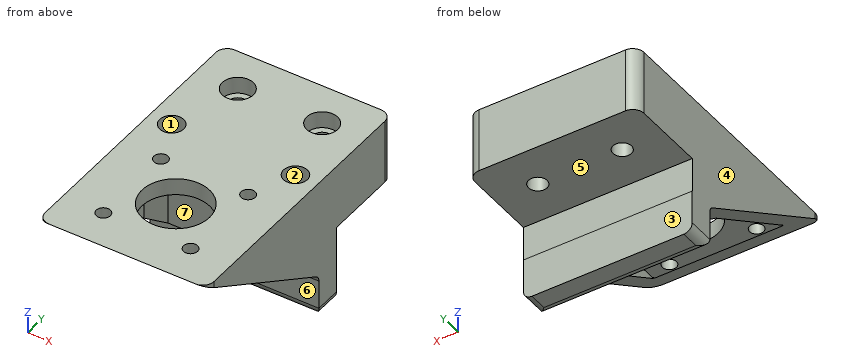
```python
from build123d import *

# Parameters (mm, degrees)
ESBO_O1_R                         = 12
ESBO_O1_R_2                       = 2.5
RESSALTO_EXTRUS_O1_DEPTH          = 6
RESSALTO_EXTRUS_O2_DEPTH          = 50
CORTE_EXTRUS_O1_DEPTH             = 61
ESBO_O5_R                         = 4.25
CORTE_EXTRUS_O2_DEPTH             = 15
REBAIXO_PARA_SHCS_M61_D           = 6.6
REBAIXO_PARA_SHCS_M61_CBORE_D     = 11
REBAIXO_PARA_SHCS_M61_CBORE_DEPTH = 6
CORTE_EXTRUS_O3_DEPTH             = 61
ESBO_O4_W                         = 60
ESBO_O4_H                         = 9.5
RESSALTO_EXTRUS_O3_DEPTH          = 15
FILETE1_R                         = 3


with BuildPart() as part:
    # Esboço1 → Ressalto-extrusão1 (new body)
    with BuildSketch(Plane.XY.offset(29.3)):
        with BuildLine():
            Line((-245.980789633, -100), (-193.980789633, -100))
            ThreePointArc((-193.980789633, -100), (-191.152362508, -98.828427125), (-189.980789633, -96))
            Line((-189.980789633, -96), (-189.980789633, -4))
            ThreePointArc((-189.980789633, -4), (-191.152362508, -1.171572875), (-193.980789633, 0))
            Line((-193.980789633, 0), (-245.980789633, 0))
            ThreePointArc((-245.980789633, 0), (-248.809216758, -1.171572875), (-249.980789633, -4))
            Line((-249.980789633, -4), (-249.980789633, -96))
            ThreePointArc((-249.980789633, -96), (-248.809216758, -98.828427125), (-245.980789633, -100))
        make_face()
        with Locations((-219.980789633, -71.15)):
            Circle(ESBO_O1_R, mode=Mode.SUBTRACT)
        with Locations((-235.480789633, -86.65)):
            Circle(ESBO_O1_R_2, mode=Mode.SUBTRACT)
        with Locations((-235.480789633, -55.65)):
            Circle(ESBO_O1_R_2, mode=Mode.SUBTRACT)
        with Locations((-204.480789633, -86.65)):
            Circle(ESBO_O1_R_2, mode=Mode.SUBTRACT)
        with Locations((-204.480789633, -55.65)):
            Circle(ESBO_O1_R_2, mode=Mode.SUBTRACT)
    extrude(amount=RESSALTO_EXTRUS_O1_DEPTH)

    # Esboço2 → Ressalto-extrusão2 (add)
    with BuildSketch(Plane(origin=(0, 0, 29.3), x_dir=(-1, 0, 0), z_dir=(0, 0, -1))):
        with BuildLine():
            Line((189.980789633, -4), (189.980789633, -96))
            ThreePointArc((189.980789633, -96), (191.152362508, -98.828427125), (193.980789633, -100))
            Line((193.980789633, -100), (245.980789633, -100))
            ThreePointArc((245.980789633, -100), (248.809216758, -98.828427125), (249.980789633, -96))
            Line((249.980789633, -96), (249.980789633, -4))
            ThreePointArc((249.980789633, -4), (248.809216758, -1.171572875), (245.980789633, 0))
            Line((245.980789633, 0), (193.980789633, 0))
            ThreePointArc((193.980789633, 0), (191.152362508, -1.171572875), (189.980789633, -4))
        make_face()
        Polygon((237.959216758, -48), (202.002362508, -48), (196.830789633, -53.171572875), (196.830789633, -89.128427125), (202.002362508, -94.3), (237.959216758, -94.3), (243.130789633, -89.128427125), (243.130789633, -53.171572875), align=None, mode=Mode.SUBTRACT)
    extrude(amount=RESSALTO_EXTRUS_O2_DEPTH)

    # Esboço3 → Corte-extrusão1 (cut, through all)
    with BuildSketch(Plane.ZY.offset(249.980789633)):
        Polygon((35.3, -100), (-20.7, -100), (-20.7, -31.056412858), (0, -31.056412858), (0, -39.485714286), align=None)
    extrude(amount=-CORTE_EXTRUS_O1_DEPTH, mode=Mode.SUBTRACT)

    # Esboço5 → Corte-extrusão2 (cut)
    with BuildSketch(Plane.XY.offset(35.3)):
        with Locations((-241.980789633, -40)):
            Circle(ESBO_O5_R)
        with Locations((-197.980789633, -40)):
            Circle(ESBO_O5_R)
    extrude(amount=-CORTE_EXTRUS_O2_DEPTH, mode=Mode.SUBTRACT)

    # Rebaixo para SHCS M61 (through all)
    with Locations(Plane.XY.offset(35.3)):
        with Locations((-234.980789633, -15), (-204.980789633, -15)):
            CounterBoreHole(REBAIXO_PARA_SHCS_M61_D / 2, REBAIXO_PARA_SHCS_M61_CBORE_D / 2, REBAIXO_PARA_SHCS_M61_CBORE_DEPTH)

    # Esboço10 → Corte-extrusão3 (cut, through all)
    with BuildSketch(Plane.ZY.offset(249.980789633)):
        Polygon((12.291276716, 1.7848e-05), (-27.708723284, 1.7848e-05), (-27.708723284, -29.999982152), (-21.235336221, -29.999982152), (-21.235336221, -31.532793492), (0, -31.532793492), (0, -29.999982152), (12.291276716, -29.999982152), align=None)
    extrude(amount=-CORTE_EXTRUS_O3_DEPTH, mode=Mode.SUBTRACT)

    # Esboço4 → Ressalto-extrusão3 (add)
    with BuildSketch(Plane(origin=(0, 0, 0), x_dir=(-1, 0, 0), z_dir=(0, 0, -1))):
        with Locations((219.980789633, -34.735714286)):
            Rectangle(ESBO_O4_W, ESBO_O4_H)
    extrude(amount=RESSALTO_EXTRUS_O3_DEPTH)

    # Filete1
    filete1_edges = [part.edges().sort_by_distance(p)[0] for p in [
        (-219.980789633, -39.485714286, 0),
        (-189.980789633, -34.735714286, -15),
        (-219.980789633, -39.485714286, -15),
        (-249.980789633, -34.735714286, -15),
    ]]
    fillet(filete1_edges, radius=FILETE1_R)


solid = part.part
```
Source: CAD feature listing. Evaluate the final solid. Frame: model axes, mm. Face numbers are marked on the shaded views. A direction names the side the tool comes from. Round coordinates to 2 decimals unless told otherwise and drop trailing zeros. Loops run counter-clockwise (first coordinate to the right, second up) from the corner with the lowest first, then second, coordinate; pieces in that order, holes last.
1. Section query C-C on y = -82. Output: boundary loops of the cut face in (x, z).
2. Section query D-D on z = 26. Output: boundary loops of the cut face in (x, y).
3. Contact query for flat-ended pins moving along their axis: pin 1 (7 mm diameter, centred on x = -241.98, y = -40, fed in from +Z); pin 2 (5.5 mm diameter, centred on x = -233.5, y = -16.5, fed in from +Z); pin 3 (6 mm diameter, centred on x = -231.5, y = -45, fed in from -Z). Output: stop coordinate, or through.
4. Section query A-A on y = -15. Output: boundary loops of the cut face in (x, z), and give its area (3 significant figures).
5. Ray query, L1, parallel to X at y = -62, z = 24; L2, parallel to X at y = -40.5, z = 24.5; L3, parallel to Y at x = -235, z = 18. Return the intervals inside material, ascending.
6. Mould query, pull axis Y, two halves, no side actions, for the marked faces 1, 2, 3 and 4. Classes: released by +Y, released by -Y, zero draft, split by the parting line, or undercut.
7. Access query for the marked faces 5, 6 and 7. Directions: +Z, -Z, +X, -X, +Y, -Y. A direction counts if a zero-diameter tool reaches every point of the face in a straight line with its end or side. Return the directions, or none.
Answers below:
1. outline: (-249.98, 24.8) - (-243.13, 24.8) - (-243.13, 29.3) - (-225.11, 29.3) - (-225.11, 35.3) - (-249.98, 35.3) - close; (-214.85, 29.3) - (-196.83, 29.3) - (-196.83, 24.8) - (-189.98, 24.8) - (-189.98, 35.3) - (-214.85, 35.3) - close
2. outline: (-249.98, -84.06) - (-243.13, -84.06) - (-243.13, -53.17) - (-237.96, -48) - (-202, -48) - (-196.83, -53.17) - (-196.83, -84.06) - (-189.98, -84.06) - (-189.98, -4) arc R4 ccw to (-193.98, 0) - (-245.98, 0) arc R4 ccw to (-249.98, -4) - close; hole circle Ø8.5 at (-241.98, -40); hole circle Ø6.6 at (-234.98, -15); hole circle Ø6.6 at (-204.98, -15); hole circle Ø8.5 at (-197.98, -40)
3. pin 1: stops at z = 20.3
3. pin 2: stops at z = 29.3
3. pin 3: stops at z = 1.47
4. outline: (-249.98, 12.29) - (-238.28, 12.29) - (-238.28, 29.3) - (-240.48, 29.3) - (-240.48, 35.3) - (-249.98, 35.3) - close; (-231.68, 12.29) - (-208.28, 12.29) - (-208.28, 29.3) - (-210.48, 29.3) - (-210.48, 35.3) - (-229.48, 35.3) - (-229.48, 29.3) - (-231.68, 29.3) - close; (-201.68, 12.29) - (-189.98, 12.29) - (-189.98, 35.3) - (-199.48, 35.3) - (-199.48, 29.3) - (-201.68, 29.3) - close
4. area: 1,020 mm2
5. L1: x = -249.98 to -243.13, -196.83 to -189.98
5. L2: x = -249.98 to -246.2, -237.76 to -202.2, -193.76 to -189.98
5. L3: y = -48 to -18.3, -11.7 to 0
6. face 1: undercut
6. face 2: undercut
6. face 3: released by +Y
6. face 4: zero draft
7. face 5: -Z, +X, -X, +Y
7. face 6: -Z, +X, -X, -Y
7. face 7: -Z, -Y
